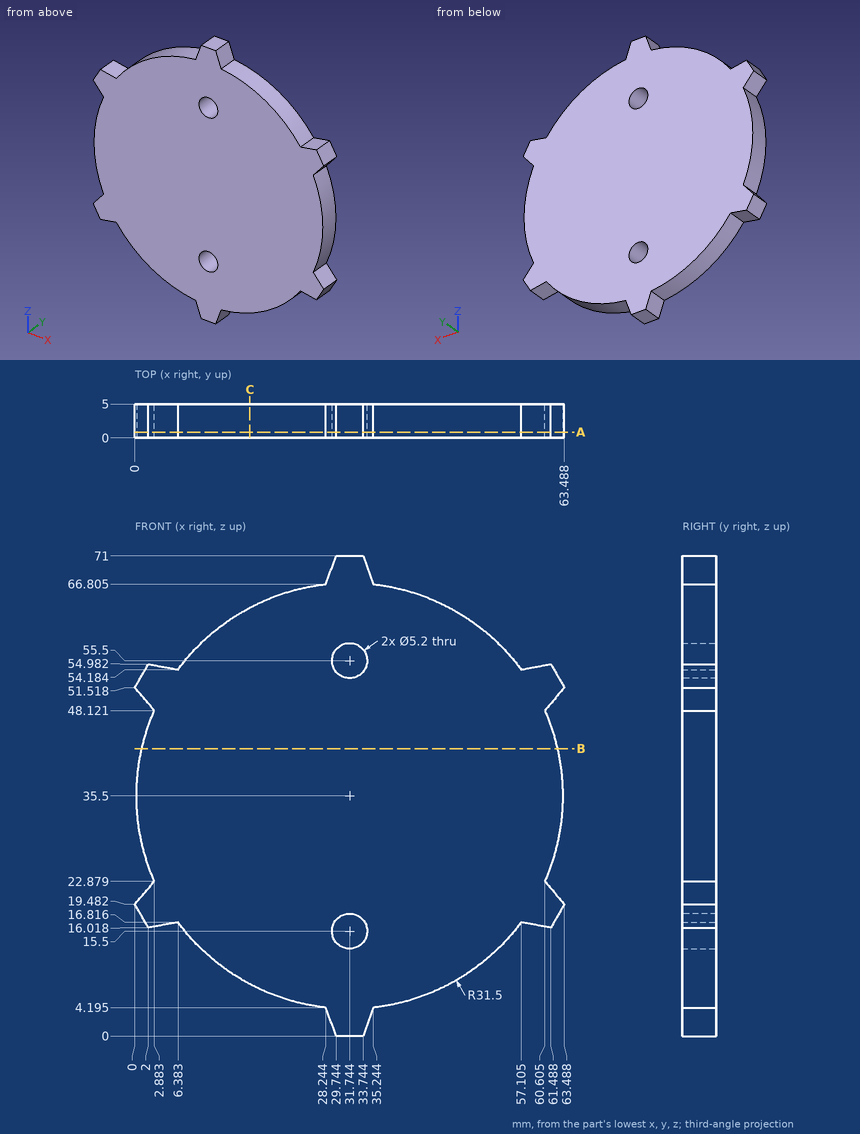
Study the drawing (mm; zero at the part's minimum x, y, z) and answer. Give positions to 0.01 mm unless a question says otherwise; leave off trailing zeros. Order: outer loops, then holes, each group sorted by start corner. A loop starts at its lowest first (then second) coordinate and runs counter-clockwise, first axis right, second up. Notation, with made-up numbers: M 63,-33.5 L 102,-33.5 A35 ccw 102,-0.5 Z; hole C 30,64.25 d10. An arc over 180 degrees is marked long. Put each result on its own line as item: value. Start each with the question number.
Item 1: Flat-ended cylindrical pins translate along their axes: P1, Ø5, axis at x = 35.5, z = 49, coming from the -Y side; P2, Ø4.5, axis at x = 31.74, z = 15.5, coming from the -Y side; P3, Ø3, axis at x = 23, y = 2, coming from the -Z side (1 decimal); P4, Ø1, axis at x = 46.5, y = 2, coming from the -Z side. Find the tip coordinate at first contact, or state that the pin passes through.
Item 2: The part is cut by section B-B, the plane z = 42.5. Determine the outline of the cut face in (x, y).
Item 3: The part is cut by section C-C, the plane x = 17. Determine the outline of the cut face in (y, z), and give its area (3 significant figures).
Item 4: Find the intervals of material crossed by line 1 along X through (y, z) = (3.45, 15.5) (1 decimal); line 2 along Z through (x, y) = (12.5, 0.75); line 3 along X through (y, z) = (4.1, 45), in increasing order.
Item 5: The part is cut by section A-A, the plane y = 0.85. Determine the outline of the cut face in (x, z) (1 decimal), and give its area (3 significant figures).
Answer key:
1. P1: stops at y = 0
1. P2: passes through
1. P3: stops at z = 4.8
1. P4: stops at z = 7.41
2. outline: M 1.03,0 L 62.46,0 L 62.46,5 L 1.03,5 Z
3. outline: M 0,7.66 L 5,7.66 L 5,63.34 L 0,63.34 Z
3. area: 278 mm²
4. line 1: x = 7.4 to 29.1, 34.3 to 56.1
4. line 2: z = 10.56 to 60.44
4. line 3: x = 1.71 to 61.78
5. outline: M 0,19.5 L 2,16 L 6.4,16.8 A31.5 ccw 28.2,4.2 L 29.7,0 L 33.7,0 L 35.2,4.2 A31.5 ccw 57.1,16.8 L 61.5,16 L 63.5,19.5 L 60.6,22.9 A31.5 ccw 60.6,48.1 L 63.5,51.5 L 61.5,55 L 57.1,54.2 A31.5 ccw 35.2,66.8 L 33.7,71 L 29.7,71 L 28.2,66.8 A31.5 ccw 6.4,54.2 L 2,55 L 0,51.5 L 2.9,48.1 A31.5 ccw 2.9,22.9 Z; hole C 31.7,15.5 d5.2; hole C 31.7,55.5 d5.2
5. area: 3,210 mm²
